```python
from build123d import *

# Parameters (mm, degrees)
BASPROSKE_W        = 5
BASPROSKE_H        = 18
TOOTHCUT_DEPTH     = 26.942243542
TEETHCUTS_COUNT    = 14
TEETHCUTS_ANGLE    = 334.285714286
BORSKE_R           = 2.5
BORE_DEPTH         = 50.0000508
BOSS_EXTRU_1_START = -5
ESQUISSE1_R        = 1.5
BOSS_EXTRU_1_DEPTH = 5


with BuildPart() as part:
    # BasProSke → Base-Revolve (revolve)
    with BuildSketch(Plane(origin=(0, 0, 0), x_dir=(1, 0, 0), z_dir=(0, 1, 0)), mode=Mode.PRIVATE) as base_revolve_sk:
        with Locations((2.5, 9)):
            Rectangle(BASPROSKE_W, BASPROSKE_H)
    revolve(base_revolve_sk.sketch.rotate(Axis((-10, 0, 0), (1, 0, 0)), 180), axis=Axis((-10, 0, 0), (1, 0, 0)))

    # TooCutSke → ToothCut (cut, through all)
    with BuildSketch(Plane(origin=(0, 0, 0), x_dir=(0, 0, -1), z_dir=(1, 0, 0))):
        with BuildLine():
            ThreePointArc((1.203681085, 12.880379812), (0, 12.9365), (-1.203681085, 12.880379812))
            ThreePointArc((-1.203681085, 12.880379812), (-1.848830306, 15.53724288), (-3.558778134, 17.670601103))
            ThreePointArc((-3.558778134, 17.670601103), (0, 18.0254), (3.558778134, 17.670601103))
            ThreePointArc((3.558778134, 17.670601103), (1.848830306, 15.53724288), (1.203681085, 12.880379812))
        make_face()
    toothcut = extrude(amount=TOOTHCUT_DEPTH, mode=Mode.SUBTRACT)

    # TeethCuts: ToothCut ×14 about axis
    teethcuts_axis = Axis((-10, 0, 0), (1, 0, 0))
    for i in range(1, TEETHCUTS_COUNT):
        add(toothcut.rotate(teethcuts_axis, i * TEETHCUTS_ANGLE / (TEETHCUTS_COUNT - 1)), mode=Mode.SUBTRACT)

    # BorSke → Bore (cut, symmetric)
    with BuildSketch(Plane(origin=(0, 0, 0), x_dir=(0, 0, -1), z_dir=(1, 0, 0))):
        with Locations(Location((0, 0, 0), (0, 0, 180))):
            Circle(BORSKE_R)
    extrude(amount=BORE_DEPTH, both=True, mode=Mode.SUBTRACT)

    # Esquisse1 → Boss.-Extru.1 (add)
    with BuildSketch(Plane(origin=(5, 0, 0), x_dir=(0, 0, -1), z_dir=(1, 0, 0)).offset(BOSS_EXTRU_1_START)):
        with BuildLine():
            Line((-5.612936991, 11.65538376), (-5.612936991, 40))
            ThreePointArc((-5.612936991, 40), (0, 45.612936991), (5.612936991, 40))
            Line((5.612936991, 40), (5.612936991, 11.65538376))
            ThreePointArc((5.612936991, 11.65538376), (0, 12.9365), (-5.612936991, 11.65538376))
        make_face()
        with Locations((0, 40)):
            Circle(ESQUISSE1_R, mode=Mode.SUBTRACT)
    extrude(amount=BOSS_EXTRU_1_DEPTH)


solid = part.part
```
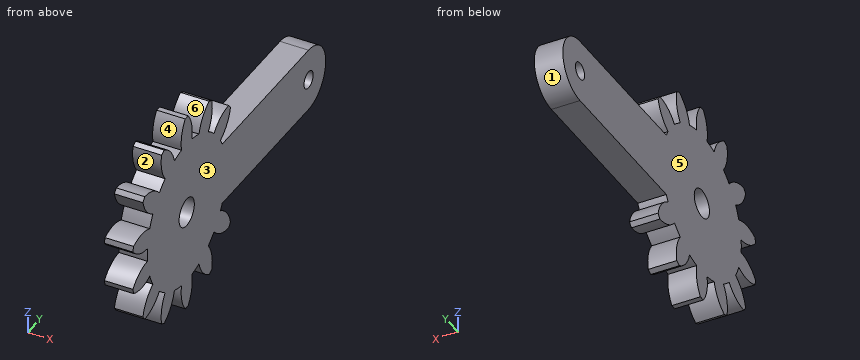
Geometry: final body of the model. Coordinates: model frame, mm. Face numbers are marked on the shaded views. A direction names the side the tool comes from. Round coordinates to 2 decimals unless told otherwise and drop trailing zeros. Write each loop counter-clockwise with the first axis right and the second up, starting at its lowest first coordinate (ties: lowest second). Pieces come first, ordered by that corner, then holes. Notation, with made-up numbers: M 39.5,-24.5 L 63.5,-24.5 A16 ccw 63.5,1.5 Z; hole C 85,-9.75 d10. An arc over 180 degrees is marked long. Answer in a Markdown table with one row per item. Add a question column.
(1) Contact query for a flat-ended pin moving along its axis: pin 1 (2.5 mm diameter, centred on x = 3.5, y = 33, fed in from -Z). Output: stop coordinate, or through.
(2) Cut plane C-C, the plane z = -15. Return the cut outline in (x, y).
(3) Cut plane B-B, the plane x = 3.85. Give the number of separate pieces and of enclosed holes in the cut face, then the cut area to 3 significant figures.
(4) Ray query, L1, parallel to Y at x = 0.85, z = 15; L2, parallel to Y at x = 2.45, z = -14; L3, parallel to Z at x = 3.5, y = 15. Return the intervals inside material, ascending.
(5) Cut plane A-A, the plane z = 0. Return the cut outline in (x, y), then the cut area to 3 significant figures.
(6) Draft query along Z for the marked faces 1, 2 and 3. Return one class per face: pulls with the +Z half, pulls with the -Z half, needs draft (parallel to the pull), parting line crosses it, or undercut.
(7) Reachability of the marked faces 4, 5 and 6 from +Z, -Z, +X, -X, +Y, -Y: full face, straight path, thin tool, end or side. Return the list, or none.
(8) Cut plane D-D, the plane y = 16. Return the cut outline in (x, z), then the cut area to 3 significant figures.
Established:
| question | item | result |
|---|---|---|
| 1 | pin 1 | z = -5.61 |
| 2 | outline | M 0,-8.38 L 5,-8.38 L 5,-5.49 L 0,-5.49 Z; M 0,-1.76 L 5,-1.76 L 5,1.76 L 0,1.76 Z; M 0,5.49 L 5,5.49 L 5,8.38 L 0,8.38 Z |
| 3 | separate pieces | 1 |
| 3 | enclosed holes | 2 |
| 3 | area | 1,040 mm² |
| 4 | L1 | -8.38 to -5.49, -1.76 to 1.76, 5.49 to 8.38 |
| 4 | L2 | -8.35 to -4.75, -1.82 to 1.82, 4.75 to 8.35 |
| 4 | L3 | -5.61 to 5.61 |
| 5 | outline | M 0,-12.94 L 5,-12.94 L 5,-2.5 L 0,-2.5 Z; M 0,2.5 L 5,2.5 L 5,38.5 L 0,38.5 Z; M 0,41.5 L 5,41.5 L 5,45.61 L 0,45.61 Z |
| 5 | area | 253 mm² |
| 6 | face 1 | parting line crosses it |
| 6 | face 2 | undercut |
| 6 | face 3 | needs draft |
| 7 | face 4 | +X, -X |
| 7 | face 5 | +Z, -Z, -X, +Y, -Y |
| 7 | face 6 | +Z, +X, -X |
| 8 | outline | M 0,-5.61 L 5,-5.61 L 5,5.61 L 0,5.61 Z |
| 8 | area | 56.1 mm² |
